```python
from build123d import *

# Parameters (mm, degrees)
BOSS_EXTRUDE1_START = -49
BOSS_EXTRUDE1_DEPTH = 5
LPATTERN1_COUNT     = 6
LPATTERN1_PITCH     = 92.4
BOSS_EXTRUDE2_START = -15
SKETCH8_W           = 10
SKETCH8_H           = 10
BOSS_EXTRUDE2_DEPTH = 330
BOSS_EXTRUDE5_REACH = 540.346
SKETCH11_W          = 10
SKETCH11_H          = 10
FILLET1_R           = 20
SKETCH12_W          = 440.103736548
SKETCH12_H          = 30
BOSS_EXTRUDE6_DEPTH = 10


with BuildPart() as part:
    # Sweep1: sweep along a path in Sketch3
    with BuildLine(Plane.XY) as sweep1_path:
        Line((0, 0), (-40, -10))
    # Sketch2 → Sweep1 (sweep)
    with BuildSketch(Plane(origin=(0, 0, 0), x_dir=(0, 0, -1), z_dir=(1, 0, 0))):
        with BuildLine():
            Line((-24.5, 0), (-22, 0))
            ThreePointArc((-22, 0), (0, -22), (22, 0))
            Line((22, 0), (24.5, 0))
            Line((24.5, 0), (24.5, -95))
            Line((24.5, -95), (-24.5, -95))
            Line((-24.5, -95), (-24.5, 0))
        make_face()
    sweep1 = sweep(path=sweep1_path.line)

    # Sketch7 → Boss-Extrude1 (add)
    with BuildSketch(Plane.XY.offset(24.5).offset(BOSS_EXTRUDE1_START)):
        Polygon((5, -70), (-445, 189.807621135), (-445, 169.807621135), (5, -90), align=None)
    extrude(amount=-BOSS_EXTRUDE1_DEPTH)

    # LPattern1: Sweep1 ×6
    with Locations(*[Vector(-0.86602540378444, 0.4999999999999978, 0) * (i * LPATTERN1_PITCH) for i in range(1, LPATTERN1_COUNT)]):
        add(sweep1)

    # Sketch8 → Boss-Extrude2 (add)
    with BuildSketch(Plane(origin=(0, 189.807621135, 0), x_dir=(1, 0, 0), z_dir=(0, 1, 0)).offset(BOSS_EXTRUDE2_START)):
        with Locations((-435.103736548, 29.5)):
            Rectangle(SKETCH8_W, SKETCH8_H)
    extrude(amount=-BOSS_EXTRUDE2_DEPTH)

    # Boss-Extrude5: up to this face of the body (flat: up to its plane)
    boss_extrude5_end = Plane(part.part.faces().sort_by_distance((-435.103736548, -155.192378865, -29.5))[0])
    # Sketch11 → Boss-Extrude5 (add, up to the picked face)
    with BuildSketch(Plane(origin=(0, -70, 0), x_dir=(1, 0, 0), z_dir=(0, 1, 0)), mode=Mode.PRIVATE) as boss_extrude5_sk1:
        with Locations((-5, 29.5)):
            Rectangle(SKETCH11_W, SKETCH11_H)
    boss_extrude5_tool1 = split(extrude(boss_extrude5_sk1.sketch, amount=-BOSS_EXTRUDE5_REACH, mode=Mode.PRIVATE), bisect_by=boss_extrude5_end, keep=Keep.BOTH, mode=Mode.PRIVATE)
    add(boss_extrude5_tool1.solids().sort_by(Axis((-5, -70, -29.5), (0, -1, 0)))[0])

    # Fillet1
    # the kernel refuses this fillet: 20 mm, written as the material it takes off along each edge
    with BuildSketch(Plane(origin=(-43.071891388, -70, -34.5), x_dir=(0, -1, 0), z_dir=(1, 0, 0))) as fillet1_piece_1:
        with BuildLine():
            CenterArc((13.228756555, -20), FILLET1_R, 90, 41.409622109)
            Line((0, -5), (-0.264575131, -4.7))
            ThreePointArc((-0.264575131, -4.7), (-0.4, -2.5), (-0.4, 0))
            Line((-0.4, 0), (0, 0.4))
            Line((0, 0.4), (13.228756555, 0.4))
            Line((13.228756555, 0.4), (13.228756555, 0))
        make_face()
    extrude(amount=76.143782777, mode=Mode.SUBTRACT)
    with BuildSketch(Plane(origin=(-397.03184516, 174.807621135, -34.5), x_dir=(0, -1, 0), z_dir=(-1, 0, 0))) as fillet1_piece_2:
        with BuildLine():
            CenterArc((13.228756555, 20), FILLET1_R, 228.590377891, 41.409622109)
            Line((0, 5), (-0.264575131, 4.7))
            ThreePointArc((-0.264575131, 4.7), (-0.4, 2.5), (-0.4, 0))
            Line((-0.4, 0), (0, -0.4))
            Line((0, -0.4), (13.228756555, -0.4))
            Line((13.228756555, -0.4), (13.228756555, 0))
        make_face()
    extrude(amount=76.143782777, mode=Mode.SUBTRACT)

    # Sketch12 → Boss-Extrude6 (add)
    with BuildSketch(Plane(origin=(0, 0, -34.5), x_dir=(-1, 0, 0), z_dir=(0, 0, -1))):
        with Locations((220.051868274, -170.192378865)):
            Rectangle(SKETCH12_W, SKETCH12_H)
    extrude(amount=-BOSS_EXTRUDE6_DEPTH)


solid = part.part
```
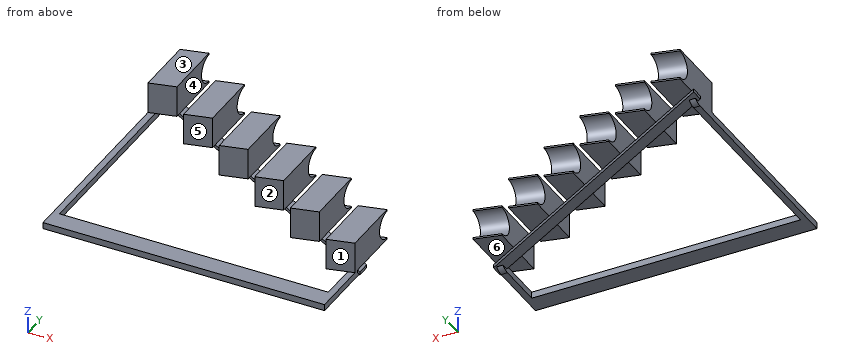
Check sheet for the modelled part. Datum: model origin and axes. Units: mm. Face numbers are marked on the shaded views. A direction names the side the tool comes from. Give positions to 0.01 mm unless a question says otherwise; leave off trailing zeros. Write each loop counter-clockwise with the first axis right and the second up, starting at its lowest first coordinate (ties: lowest second). Pieces come first, ordered by that corner, then holes.
Item 1: Access from +Z, -Z, +X, -X, +Y, -Y to the whole of each face (thin tool, end or side, straight path). Record for the marked faces 4, 5 and 6.
Item 2: Gauge pin test, flat ends, axial feed: pin 1 (1.5 mm diameter, centred on x = -276.5, z = 10.5, fed in from -Y); pin 2 (3 mm diameter, centred on y = 32, z = -31.5, fed in from +X); pin 3 (20 mm diameter, centred on x = -264, y = 58, fed in from -Z). Record the tip position at first contact, or that the pin passes through.
Item 3: Cross-section at A-A (x = -130). Enter the section's corners in (y, z).
Item 4: Scan lines: L1, parallel to X at y = 74, z = -22.5; L2, parallel to X at y = -63.5, z = 16.5; L3, parallel to Y at x = -238, z = -27. Record each from-to range of solid material in increasing order.
Item 5: Cross-section at B-B (z = 12). Count the separate pieces of the cut face and the enclosed holes in it, and give its area (3 significant figures).
Item 6: Draft check along X on the marked faces 1, 2 and 3. Enter one of: released by +X, released by -X, zero draft, split by the parting line, or undercut.
Report:
1. face 4: +Z, +Y, -Y
1. face 5: +Z, -Z, -Y
1. face 6: -Z, +X, +Y
2. pin 1: stops at y = 34.3
2. pin 2: stops at x = -430.1
2. pin 3: stops at z = -29.5
3. outline: (-185.19, -34.5) - (-155.19, -34.5) - (-155.19, -24.5) - (-185.19, -24.5) - close; (-12.06, -29.5) - (7.94, -29.5) - (7.94, -24.5) - (-12.06, -24.5) - close
4. L1: x = -280.06 to -240.06, -200.04 to -160.04
4. L2: x = -40 to 0
4. L3: y = -185.19 to -155.19, 50.3 to 70.3
5. separate pieces: 6
5. enclosed holes: 0
5. area: 18,400 mm2
6. face 1: released by +X
6. face 2: undercut
6. face 3: zero draft
